```python
from build123d import *

# Parameters (mm, degrees)
SKETCH1_W                = 75
SKETCH1_H                = 35
BOSS_EXTRUDE1_DEPTH      = 5
SKETCH2_R                = 2
BOSS_EXTRUDE2_DEPTH      = 10
SKETCH3_W                = 75
SKETCH3_H                = 35
BOSS_EXTRUDE3_DEPTH      = 15
CUT_EXTRUDE2_DEPTH       = 10
SKETCH8_W                = 12.55
SKETCH8_H                = 5
SKETCH8_H_2              = 2.55
BOSS_EXTRUDE6_DEPTH      = 4.57
SKETCH9_R                = 2.1
CUT_EXTRUDE3_DEPTH       = 4.57
SKETCH14_W               = 3
SKETCH14_H               = 10
CUT_EXTRUDE5_DEPTH       = 17
SKETCH15_R               = 2.75
CUT_EXTRUDE6_DEPTH       = 1.5
FILLET1_R                = 1
CUT_EXTRUDE7_START       = -5
SKETCH19_R               = 2
CUT_EXTRUDE7_DEPTH       = 5
SKETCH20_W               = 6.17
SKETCH20_H               = 24
BOSS_EXTRUDE7_DEPTH      = 12
SKETCH21_W               = 6.17
SKETCH21_H               = 24
BOSS_EXTRUDE8_DEPTH      = 12
SKETCH24_R               = 2.1
CUT_EXTRUDE8_DEPTH       = 60.774520492
SKETCH25_R               = 4
CUT_EXTRUDE9_DEPTH       = 2
BOSS_EXTRUDE10_DEPTH     = 41
CUT_EXTRUDE11_DEPTH      = 99.402819573
CUT_EXTRUDE11_DEPTH_BACK = 99.402819573
SKETCH30_R               = 2.1
FILLET2_R                = 6.2
SKETCH31_W               = 15
SKETCH31_H               = 15
BOSS_EXTRUDE11_DEPTH     = 10
SKETCH32_W               = 5
SKETCH32_H               = 12
CUT_EXTRUDE12_DEPTH      = 10
SKETCH34_W               = 3.2
SKETCH34_H               = 3.2
CUT_EXTRUDE13_DEPTH      = 28
CUT_EXTRUDE14_START      = -5
SKETCH35_R               = 2
CUT_EXTRUDE14_DEPTH      = 5


with BuildPart() as part:
    # Sketch1 → Boss-Extrude1 (new body)
    with BuildSketch(Plane.XY):
        Rectangle(SKETCH1_W, SKETCH1_H)
    extrude(amount=BOSS_EXTRUDE1_DEPTH)

    # Sketch2 → Boss-Extrude2 (add)
    with BuildSketch(Plane.XY.offset(5)):
        with Locations(Location((-14.2, 0.5, 0), (0, 0, 180))):
            Circle(SKETCH2_R)
        with Locations(Location((14.2, 0.5, 0), (0, 0, 180))):
            Circle(SKETCH2_R)
    extrude(amount=BOSS_EXTRUDE2_DEPTH)

    # Sketch3 → Boss-Extrude3 (add)
    with BuildSketch(Plane(origin=(0, 0, 0), x_dir=(-1, 0, 0), z_dir=(0, 0, -1))):
        Polygon((40.5, 20.5), (-37.5, 20.5), (-40.5, 20.5), (-40.5, -20.5), (40.5, -20.5), (40.5, -17.5), align=None)
        Rectangle(SKETCH3_W, SKETCH3_H, mode=Mode.SUBTRACT)
    extrude(amount=-BOSS_EXTRUDE3_DEPTH)

    # Sketch4 → Cut-Extrude2 (cut)
    with BuildSketch(Plane(origin=(0, 20.5, 0), x_dir=(1, 0, 0), z_dir=(0, 1, 0))):
        Polygon((-37.5, -5), (-37.5, -12.5), (-37.5, -14), (-37.5, -15), (37.5, -15), (37.5, -14), (37.5, -12.5), (37.5, -5), align=None)
    extrude(amount=-CUT_EXTRUDE2_DEPTH, mode=Mode.SUBTRACT)

    # Sketch8 → Boss-Extrude6 (add)
    with BuildSketch(Plane(origin=(0, 20.5, 0), x_dir=(1, 0, 0), z_dir=(0, 1, 0))):
        Polygon((0, -15), (0, -5), (-12.55, -5), (-12.55, -22.55), (0, -22.55), align=None)
        Polygon((12.55, -5), (0, -5), (0, -15), (0, -22.55), (12.55, -22.55), align=None)
        with Locations((-6.275, -2.5)):
            Rectangle(SKETCH8_W, SKETCH8_H)
        with Locations((-6.275, 1.275)):
            Rectangle(SKETCH8_W, SKETCH8_H_2)
        with Locations((6.275, 1.275)):
            Rectangle(SKETCH8_W, SKETCH8_H_2)
        with Locations((6.275, -2.5)):
            Rectangle(SKETCH8_W, SKETCH8_H)
    extrude(amount=BOSS_EXTRUDE6_DEPTH)

    # Sketch9 → Cut-Extrude3 (cut)
    with BuildSketch(Plane(origin=(0, 25.07, 0), x_dir=(1, 0, 0), z_dir=(0, 1, 0))):
        with Locations(Location((0, -10, 0), (0, 0, 270))):
            Circle(SKETCH9_R)
        with Locations(Location((-6.349818895, -3.650181105, 0), (0, 0, 270))):
            Circle(SKETCH9_R)
        with Locations(Location((6.349818895, -3.650181105, 0), (0, 0, 270))):
            Circle(SKETCH9_R)
        with Locations(Location((6.349818895, -16.349818895, 0), (0, 0, 270))):
            Circle(SKETCH9_R)
        with Locations(Location((-6.349818895, -16.349818895, 0), (0, 0, 270))):
            Circle(SKETCH9_R)
    extrude(amount=-CUT_EXTRUDE3_DEPTH, mode=Mode.SUBTRACT)

    # Sketch14 → Cut-Extrude5 (cut)
    with BuildSketch(Plane(origin=(0, 20.5, 0), x_dir=(1, 0, 0), z_dir=(0, 1, 0))):
        with Locations((-39, -10)):
            Rectangle(SKETCH14_W, SKETCH14_H)
        with Locations((39, -10)):
            Rectangle(SKETCH14_W, SKETCH14_H)
    extrude(amount=-CUT_EXTRUDE5_DEPTH, mode=Mode.SUBTRACT)

    # Sketch15 → Cut-Extrude6 (cut)
    with BuildSketch(Plane(origin=(0, 20.5, 0), x_dir=(1, 0, 0), z_dir=(0, 1, 0))):
        with Locations((-6.349818895, -3.650181105)):
            Circle(SKETCH15_R)
        with Locations((6.349818895, -3.650181105)):
            Circle(SKETCH15_R)
    extrude(amount=-CUT_EXTRUDE6_DEPTH, mode=Mode.SUBTRACT)

    # Fillet1
    fillet1_edges = [part.edges().sort_by_distance(p)[0] for p in [
        (-8.745750645, 19.75, 5),
        (-3.953887145, 19.75, 5),
        (3.953887145, 19.75, 5),
        (8.745750645, 19.75, 5),
    ]]
    fillet(fillet1_edges, radius=FILLET1_R)

    # Sketch19 → Cut-Extrude7 (cut)
    with BuildSketch(Plane.XY.offset(15).offset(CUT_EXTRUDE7_START)):
        with Locations(Location((-14.2, 0.5, 0), (0, 0, 180))):
            Circle(SKETCH19_R)
    extrude(amount=CUT_EXTRUDE7_DEPTH, mode=Mode.SUBTRACT)

    # Sketch20 → Boss-Extrude7 (add)
    with BuildSketch(Plane(origin=(40.5, 0, 0), x_dir=(0, 0, -1), z_dir=(1, 0, 0))):
        with Locations((-11.915, -8.5)):
            Rectangle(SKETCH20_W, SKETCH20_H)
    extrude(amount=BOSS_EXTRUDE7_DEPTH)

    # Sketch21 → Boss-Extrude8 (add)
    with BuildSketch(Plane.ZY.offset(40.5)):
        with Locations((11.915, -8.5)):
            Rectangle(SKETCH21_W, SKETCH21_H)
    extrude(amount=BOSS_EXTRUDE8_DEPTH)

    # Sketch24 → Cut-Extrude8 (cut, through all)
    with BuildSketch(Plane(origin=(0, 0, 8.83), x_dir=(-1, 0, 0), z_dir=(0, 0, -1))):
        with Locations(Location((-46.5, -3.5, 0), (0, 0, 90))):
            Circle(SKETCH24_R)
        with Locations(Location((-46.5, -13.5, 0), (0, 0, 90))):
            Circle(SKETCH24_R)
        with Locations(Location((46.5, -3.5, 0), (0, 0, 90))):
            Circle(SKETCH24_R)
        with Locations(Location((46.5, -13.5, 0), (0, 0, 90))):
            Circle(SKETCH24_R)
    extrude(amount=-CUT_EXTRUDE8_DEPTH, mode=Mode.SUBTRACT)

    # Sketch25 → Cut-Extrude9 (cut)
    with BuildSketch(Plane.XY.offset(15)):
        with Locations((-46.5, -3.5)):
            Circle(SKETCH25_R)
        with Locations((-46.5, -13.5)):
            Circle(SKETCH25_R)
        with Locations((46.5, -13.5)):
            Circle(SKETCH25_R)
        with Locations((46.5, -3.5)):
            Circle(SKETCH25_R)
    extrude(amount=-CUT_EXTRUDE9_DEPTH, mode=Mode.SUBTRACT)

    # Sketch28 → Boss-Extrude10 (add)
    with BuildSketch(Plane.XZ.offset(20.5)):
        Polygon((-25.5, 0), (-42.57, 0), (-42.57, -29.4), (-38, -29.4), (-38, -4), (-25.5, -4), align=None)
        Polygon((25.5, 0), (42.57, 0), (42.57, -29.4), (38, -29.4), (38, -4), (25.5, -4), align=None)
    extrude(amount=-BOSS_EXTRUDE10_DEPTH)

    # Sketch30 → Cut-Extrude11 (cut, two sides: drawn at the far end of the back side and taken through both)
    with BuildSketch(Plane(origin=(-38, 0, 0), x_dir=(0, 0, -1), z_dir=(1, 0, 0)).offset(-CUT_EXTRUDE11_DEPTH_BACK)):
        with Locations(Location((23.2, 0, 0), (0, 0, 180))):
            Circle(SKETCH30_R)
        with Locations(Location((23.2, 12.7, 0), (0, 0, 180))):
            Circle(SKETCH30_R)
        with Locations(Location((23.2, -12.7, 0), (0, 0, 180))):
            Circle(SKETCH30_R)
    extrude(amount=CUT_EXTRUDE11_DEPTH + CUT_EXTRUDE11_DEPTH_BACK, mode=Mode.SUBTRACT)

    # Fillet2
    # the kernel refuses this fillet: 6.2 mm, written as the material it takes off along each edge
    with BuildSketch(Plane(origin=(12.55, 5, 22.55), x_dir=(0, 0, -1), z_dir=(0, 1, 0))) as fillet2_piece_1:
        with BuildLine():
            CenterArc((FILLET2_R, FILLET2_R), FILLET2_R, 180, 90)
            Line((0, FILLET2_R), (0, 0))
            Line((0, 0), (FILLET2_R, 0))
        make_face()
    extrude(amount=35.57, mode=Mode.SUBTRACT)
    with BuildSketch(Plane(origin=(12.55, 20.5, -2.55), x_dir=(0, 0, 1), z_dir=(0, 1, 0))) as fillet2_piece_2:
        with BuildLine():
            CenterArc((FILLET2_R, -FILLET2_R), FILLET2_R, 90, 90)
            Line((0, -FILLET2_R), (0, 0))
            Line((0, 0), (FILLET2_R, 0))
        make_face()
    extrude(amount=20.07, mode=Mode.SUBTRACT)
    with BuildSketch(Plane(origin=(-12.55, 20.5, -2.55), x_dir=(0, 0, 1), z_dir=(0, 1, 0))) as fillet2_piece_3:
        with BuildLine():
            CenterArc((FILLET2_R, FILLET2_R), FILLET2_R, 180, 90)
            Line((0, FILLET2_R), (0, 0))
            Line((0, 0), (FILLET2_R, 0))
        make_face()
    extrude(amount=20.07, mode=Mode.SUBTRACT)
    with BuildSketch(Plane(origin=(-12.55, 5, 22.55), x_dir=(0, 0, -1), z_dir=(0, 1, 0))) as fillet2_piece_4:
        with BuildLine():
            CenterArc((FILLET2_R, -FILLET2_R), FILLET2_R, 90, 90)
            Line((0, -FILLET2_R), (0, 0))
            Line((0, 0), (FILLET2_R, 0))
        make_face()
    extrude(amount=35.57, mode=Mode.SUBTRACT)

    # Sketch31 → Boss-Extrude11 (add)
    with BuildSketch(Plane.XZ.offset(20.5)):
        with Locations((0, 7.5)):
            Rectangle(SKETCH31_W, SKETCH31_H)
    extrude(amount=BOSS_EXTRUDE11_DEPTH)

    # Sketch32 → Cut-Extrude12 (cut)
    with BuildSketch(Plane.XZ.offset(30.5)):
        with Locations((0, 7.5)):
            Rectangle(SKETCH32_W, SKETCH32_H)
    extrude(amount=-CUT_EXTRUDE12_DEPTH, mode=Mode.SUBTRACT)

    # Sketch34 → Cut-Extrude13 (cut)
    with BuildSketch(Plane.ZY.offset(7.5)):
        with Locations((7.5, -25.5)):
            Rectangle(SKETCH34_W, SKETCH34_H)
    extrude(amount=-CUT_EXTRUDE13_DEPTH, mode=Mode.SUBTRACT)

    # Sketch35 → Cut-Extrude14 (cut)
    with BuildSketch(Plane.XY.offset(15).offset(CUT_EXTRUDE14_START)):
        with Locations(Location((14.2, 0.5, 0), (0, 0, 180))):
            Circle(SKETCH35_R)
    extrude(amount=CUT_EXTRUDE14_DEPTH, mode=Mode.SUBTRACT)


solid = part.part
```
Could you check a few things on this model? Use its own coordinates, in mm. A direction names the side the tool comes from. Coordinates: 2 decimals unless noted, no trailing zeros. Loops run counter-clockwise (first coordinate to the right, second up) from the corner with the lowest first, then second, coordinate; pieces in that order, holes last.
1) Please list where these lines run through material, in increasing order: line 1 along X through (y, z) = (-3.5, 10.6); line 2 along Y through (x, z) = (-39.95, -23.2); line 3 along X through (y, z) = (1.5, 12).
Reported:
line 1: x = -52.5 to -48.6, -44.4 to -37.5, 37.5 to 44.4, 48.6 to 52.5
line 2: y = -20.5 to -14.8, -10.6 to -2.1, 2.1 to 10.6, 14.8 to 20.5
line 3: x = -52.5 to -37.5, 37.5 to 52.5
2) Will these pins go through, and if not, where does the flat tip stop? pin 1 Ø1.6 at (x, y) = (-6, -26) entering from -Z; pin 2 Ø3.5 at (x, z) = (0, 10) entering from +Y; pin 3 Ø3 at (x, y) = (-32.5, -18) entering from +Z.
Reported:
pin 1: stops at z = 0
pin 2: stops at y = -17.5
pin 3: stops at z = 15
3) Imagine slicing it at D-D (x = -33). List the corners of the cut face in (y, z) for me.
Reported:
outline: (-20.5, -4) - (20.5, -4) - (20.5, 5) - (-17.5, 5) - (-17.5, 15) - (-20.5, 15) - close
4) Imagine slicing it at A-A (x = 0). List the corners of the cut face in (y, z) for me.
Reported:
outline: (-30.5, 0) - (20.5, 0) - (20.5, -2.55) - (25.07, -2.55) - (25.07, 7.9) - (20.5, 7.9) - (20.5, 5) - (-17.5, 5) - (-17.5, 15) - (-30.5, 15) - (-30.5, 13.5) - (-20.5, 13.5) - (-20.5, 1.5) - (-30.5, 1.5) - close; (20.5, 12.1) - (25.07, 12.1) - (25.07, 22.55) - (20.5, 22.55) - close
5) Imagine slicing it at B-B (y = 7). List the corners of the cut face in (x, z) for me, and give its area (3 significant figures).
Reported:
outline: (-42.57, -29.4) - (-38, -29.4) - (-38, -4) - (-25.5, -4) - (-25.5, 0) - (25.5, 0) - (25.5, -4) - (38, -4) - (38, -29.4) - (42.57, -29.4) - (42.57, 0) - (40.5, 0) - (40.5, 5) - (-40.5, 5) - (-40.5, 0) - (-42.57, 0) - close
area: 774 mm2
6) Which directions (+Z, -Z, +X, -X, +Y, -Y) give clear straight access to the entire face, cutting with the end or side of a thin tool? Please do faces 4 (the face through (42.504, -13.324, 14.014)), 5 (the face through (-5, -23.9, 7)), 6 (the face through (8.432, 22.817, 16.076)), 7 (the face through (-46, -9, 8.83)).
Reported:
face 4: +Z
face 5: +X, -X
face 6: +Y
face 7: -X, +Y, -Y
7) Imagine slicing it at C-C (x = -46.5). List the corners of the cut face in (y, z) for me, and give its area (3 significant figures).
Reported:
outline: (-20.5, 8.83) - (-15.6, 8.83) - (-15.6, 13) - (-17.5, 13) - (-17.5, 15) - (-20.5, 15) - close; (-11.4, 8.83) - (-5.6, 8.83) - (-5.6, 13) - (-7.5, 13) - (-7.5, 15) - (-9.5, 15) - (-9.5, 13) - (-11.4, 13) - close; (-1.4, 8.83) - (3.5, 8.83) - (3.5, 15) - (0.5, 15) - (0.5, 13) - (-1.4, 13) - close
area: 81.1 mm2
8) Thinking about a two-plate mould opening in X: for faces 1 (the face through (-16.047, 1.266, 7.465)), 2 (the face through (30, -20.5, 3)), 3 (the face through (12.55, 23, 10)), which applies, released by +X, released by -X, zero draft, split by the parting line, or undercut?
Reported:
face 1: undercut
face 2: zero draft
face 3: released by +X
